Geometry: final body of the model. Coordinates: model frame, mm. A direction names the side the tool comes from. Give positions to 0.01 mm unless a question says otherwise; leave off trailing zeros. Write each loop counter-clockwise with the first axis right and the second up, starting at its lowest first coordinate (ties: lowest second). Pieces come first, ordered by that corner, then holes. Notation, with made-up numbers: (14.5, 75.25) - (20.5, 75.25) arc R16 ccw to (20.5, 100.25) - close; hole circle Ø2 at (65.5, 74.25). An arc over 180 degrees is marked (long way). Return JSON: item names as keys, results as strings.
from build123d import *

# Parameters (mm, degrees)
SKETCH1_R           = 60
BOSS_EXTRUDE1_DEPTH = 10
SKETCH2_R           = 11
CUT_EXTRUDE1_DEPTH  = 7
SKETCH3_R           = 7.5
CUT_EXTRUDE2_DEPTH  = 86.141059425
SKETCH5_R           = 4.975
SKETCH5_R_2         = 2.05
CUT_EXTRUDE4_DEPTH  = 86.440037453
SKETCH6_R           = 2.05
CUT_EXTRUDE5_DEPTH  = 86.440037453
CIRPATTERN1_COUNT   = 4
SKETCH7_R           = 17.5
CUT_EXTRUDE6_DEPTH  = 86.440037453


with BuildPart() as part:
    # Sketch1 → Boss-Extrude1 (new body)
    with BuildSketch(Plane(origin=(0, 0, 0), x_dir=(1, 0, 0), z_dir=(0, 1, 0))):
        with Locations(Location((0, 0, 0), (0, 0, 270))):
            Circle(SKETCH1_R)
    extrude(amount=BOSS_EXTRUDE1_DEPTH)

    # Sketch2 → Cut-Extrude1 (cut)
    with BuildSketch(Plane(origin=(0, 10, 0), x_dir=(1, 0, 0), z_dir=(0, 1, 0))):
        with Locations(Location((0, -33, 0), (0, 0, 270))):
            Circle(SKETCH2_R)
    extrude(amount=-CUT_EXTRUDE1_DEPTH, mode=Mode.SUBTRACT)

    # Sketch3 → Cut-Extrude2 (cut, through all)
    with BuildSketch(Plane(origin=(0, 3, 0), x_dir=(1, 0, 0), z_dir=(0, 1, 0))):
        with Locations(Location((0, -33, 0), (0, 0, 270))):
            Circle(SKETCH3_R)
    extrude(amount=-CUT_EXTRUDE2_DEPTH, mode=Mode.SUBTRACT)

    # Sketch5 → Cut-Extrude4 (cut, through all)
    with BuildSketch(Plane(origin=(0, 10, 0), x_dir=(1, 0, 0), z_dir=(0, 1, 0))):
        with Locations(Location((-33.587572106, -33.587572106, 0), (0, 0, 270))):
            Circle(SKETCH5_R)
        with Locations(Location((-43.487067043, -23.68807717, 0), (0, 0, 270))):
            Circle(SKETCH5_R_2)
        with Locations(Location((-23.68807717, -43.487067043, 0), (0, 0, 270))):
            Circle(SKETCH5_R_2)
    cut_extrude4 = extrude(amount=-CUT_EXTRUDE4_DEPTH, mode=Mode.SUBTRACT)

    # Sketch6 → Cut-Extrude5 (cut, through all)
    with BuildSketch(Plane(origin=(0, 10, 0), x_dir=(1, 0, 0), z_dir=(0, 1, 0))):
        with Locations(Location((0, -49.52, 0), (0, 0, 270))):
            Circle(SKETCH6_R)
    cut_extrude5 = extrude(amount=-CUT_EXTRUDE5_DEPTH, mode=Mode.SUBTRACT)

    # CirPattern1: Cut-Extrude4, Cut-Extrude5 ×4 about axis
    cirpattern1_axis = Axis((0, 0, 0), (0, 1, 0))
    add([cut_extrude4.rotate(cirpattern1_axis, i * 360 / CIRPATTERN1_COUNT) for i in range(1, CIRPATTERN1_COUNT)], mode=Mode.SUBTRACT)
    add([cut_extrude5.rotate(cirpattern1_axis, i * 360 / CIRPATTERN1_COUNT) for i in range(1, CIRPATTERN1_COUNT)], mode=Mode.SUBTRACT)

    # Sketch7 → Cut-Extrude6 (cut, through all)
    with BuildSketch(Plane(origin=(0, 10, 0), x_dir=(1, 0, 0), z_dir=(0, 1, 0))):
        with Locations(Location((0, 0, 0), (0, 0, 270))):
            Circle(SKETCH7_R)
    extrude(amount=-CUT_EXTRUDE6_DEPTH, mode=Mode.SUBTRACT)


solid = part.part
Q1. Pin query (flat end, axial travel): P1, Ø1, axis at y = 5, z = -43.5, coming from the +X side; P2, Ø1.5, axis at y = 8.5, z = 1, coming from the -X side; P3, Ø19.5, axis at x = 0, z = 33, coming from the +Y side. Return the tip coordinate at first contact, or that it passes through.
Answer key:
{"P1": "stops at x = 41.84", "P2": "stops at x = -60", "P3": "stops at y = 3"}
Q2. Section query A-A, the plane x = 0. Return the cut outline in (y, z).
Answer key:
{"outline": "(0, -60) - (10, -60) - (10, -51.57) - (0, -51.57) - close; (0, -47.47) - (10, -47.47) - (10, -17.5) - (0, -17.5) - close; (0, 17.5) - (10, 17.5) - (10, 22) - (3, 22) - (3, 25.5) - (0, 25.5) - close; (0, 40.5) - (3, 40.5) - (3, 44) - (10, 44) - (10, 47.47) - (0, 47.47) - close; (0, 51.57) - (10, 51.57) - (10, 60) - (0, 60) - close"}
Q3. Mould query, pull axis Z, two halves, no side actions, for faces 3 (the cylindrical face through (0.33, 1.521, 25.507)), 4 (the cylindrical face through (2.64, 4.93, -59.94)), 5 (the cylindrical face through (-41.76, 5.07, 24.79)), 6 (the flat face through (-12.5, 10, 12.5)). Classes: pulls with the +Z half, pulls with the -Z half, needs draft (parallel to the pull), parting line crosses it, or undercut.
Answer key:
{"face 3": "undercut", "face 4": "parting line crosses it", "face 5": "undercut", "face 6": "needs draft"}
Q4. Section query C-C, the plane x = -49.52. Return the cut outline in (y, z).
Answer key:
{"outline": "(0, -33.88) - (10, -33.88) - (10, -2.05) - (0, -2.05) - close; (0, 2.05) - (10, 2.05) - (10, 33.88) - (0, 33.88) - close"}
Q5. Material intervals for probe 1 along Z at (x, y) = (-30.5, 4.5); probe 2 along Z at (x, y) = (45, 3.25); probe 3 along X at (y, z) = (5, 33), sorted ascending. Write a range as [from, to].
Answer key:
{"probe 1": "z = [-51.67, -37.49], [-29.69, 29.69], [37.49, 51.67]", "probe 2": "z = [-39.69, -25.07], [-22.3, 22.3], [25.07, 39.69]", "probe 3": "x = [-50.11, -38.53], [-28.65, -11], [11, 28.65], [38.53, 50.11]"}
Q6. Set-up query: faces 1 (the cylindrical face through (-9.759, 6.549, 38.076)), 2 (the cylindrical face through (47.47, 5.07, -0.09)). Return all of +Z, -Z, +X, -X, +Y, -Y with unobstructed straight access to the full face (end or side cutting, diameter ignored); none if empty.
Answer key:
{"face 1": "+Y", "face 2": "+Y, -Y"}
Q7. Section query B-B, the plane z = 0. Return the cut outline in (x, y).
Answer key:
{"outline": "(-60, 0) - (-51.57, 0) - (-51.57, 10) - (-60, 10) - close; (-47.47, 0) - (-17.5, 0) - (-17.5, 10) - (-47.47, 10) - close; (17.5, 0) - (47.47, 0) - (47.47, 10) - (17.5, 10) - close; (51.57, 0) - (60, 0) - (60, 10) - (51.57, 10) - close"}
Q8. Section query D-D, the plane z = 49.52. Return the cut outline in (x, y), plus the area to 3 significant figures.
Answer key:
{"outline": "(-33.88, 0) - (-2.05, 0) - (-2.05, 10) - (-33.88, 10) - close; (2.05, 0) - (33.88, 0) - (33.88, 10) - (2.05, 10) - close", "area": "637 mm^2"}
